Could you check a few things on this model? Use its own coordinates, in mm. Face numbers are marked on the shaded views. A direction names the side the tool comes from. Give positions to 0.01 mm unless a question says otherwise; leave off trailing zeros. Order: outer loops, then holes, each group sorted by start corner. A loop starts at its lowest first (then second) coordinate and runs counter-clockwise, first axis right, second up.
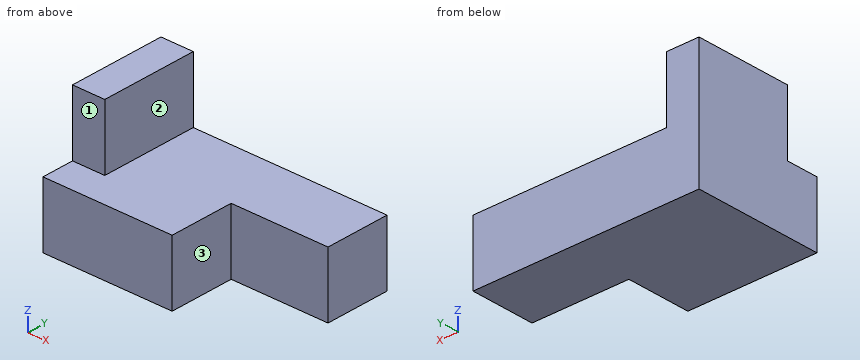
from build123d import *

# Parameters (mm, degrees)
F0_W     = 25.4
F0_H     = 25.4
F1_DEPTH = 12.7
F2_W     = 6.35
F2_H     = 19.05
F3_DEPTH = 12.7
F4_W     = 12.7
F4_H     = 12.7
F5_DEPTH = 19.05


with BuildPart() as f1:
    # F0 (on Top) → F1 (new body)
    with BuildSketch(Plane.XY):
        with Locations((12.7, -12.7)):
            Rectangle(F0_W, F0_H)
    extrude(amount=F1_DEPTH)

    # F2 (on face) → F3 (join)
    with BuildSketch(Plane.XY.offset(12.7)):
        with Locations((3.175, -9.525)):
            Rectangle(F2_W, F2_H)
    extrude(amount=F3_DEPTH)

    # F4 (on face) → F5 (join)
    with BuildSketch(Plane.YZ.offset(25.4)):
        with Locations((-6.35, 6.35)):
            Rectangle(F4_W, F4_H)
    extrude(amount=F5_DEPTH)


solid = f1.part
Item 1: Imagine slicing it at B-B on x = 4.5. List the corners of the cut face in (y, z) for me, then the cut area to 3 significant figures.
Findings:
outline: (-25.4, 0) - (0, 0) - (0, 25.4) - (-19.05, 25.4) - (-19.05, 12.7) - (-25.4, 12.7) - close
area: 565 mm2
Item 2: Imagine slicing it at A-A on y = -6.5. List the corners of the cut face in (x, z) for me.
Findings:
outline: (0, 0) - (44.45, 0) - (44.45, 12.7) - (6.35, 12.7) - (6.35, 25.4) - (0, 25.4) - close
Item 3: Imagine slicing it at C-C on z = 22.75. List the corners of the cut face in (x, y) for me, then the cut area to 3 significant figures.
Findings:
outline: (0, -19.05) - (6.35, -19.05) - (6.35, 0) - (0, 0) - close
area: 121 mm2
Item 4: Imagine slicing it at D-D on x = 40.5. List the corners of the cut face in (y, z) for me, then the cut area to 3 significant figures.
Findings:
outline: (-12.7, 0) - (0, 0) - (0, 12.7) - (-12.7, 12.7) - close
area: 161 mm2
Item 5: For pin 1 (6.5 mm diameter, centred on x = 31, z = 3.5, fed in from -Y); pin 2 (8 mm diameter, centred on x = 17, z = 19.5, fed in from +Y); pin 3 (7 mm diameter, centred on x = 3.5, z = 18.5, fed in from -Y); pin 4 (12.5 mm diameter, centred on x = 24.5, y = -6.5, fed in from +Z), each with a flat end and sliding along its axis, tell me the tip position at first contact or that it passes through.
Findings:
pin 1: stops at y = -12.7
pin 2: passes through
pin 3: stops at y = -19.05
pin 4: stops at z = 12.7
Item 6: Please list where these lines run through material, in increasing order: line 1 along Y through (x, z) = (28, 10.75); line 2 along Z through (x, y) = (30.5, -5); line 3 along X through (y, z) = (-20, 5).
Findings:
line 1: y = -12.7 to 0
line 2: z = 0 to 12.7
line 3: x = 0 to 25.4
Item 7: For the marked faces 1, 2 and 3, which set-ups out of +Z, -Z, +X, -X, +Y, -Y let a thin tool reach every point of the face, with its end or its side?
Findings:
face 1: +Z, +X, -X, -Y
face 2: +Z, +X, +Y, -Y
face 3: +Z, -Z, +X, -Y
